Verification items for this drawing (mm, ordinates from the low corner). Round coordinates to 2 decimals unless told otherwise and drop trailing zeros. Order: outer loops, then holes, each group sorted by start corner. A loop starts at its lowest first (then second) coordinate and runs counter-clockwise, first axis right, second up. Notation, with made-up numbers: (-31, 11) - (-7, 11) arc R18 ccw to (-7, 26) - close; hole circle Ø8 at (59, 48). An arc over 180 degrees is marked (long way). Answer as CSV lines item,"result". Start each with the question number.
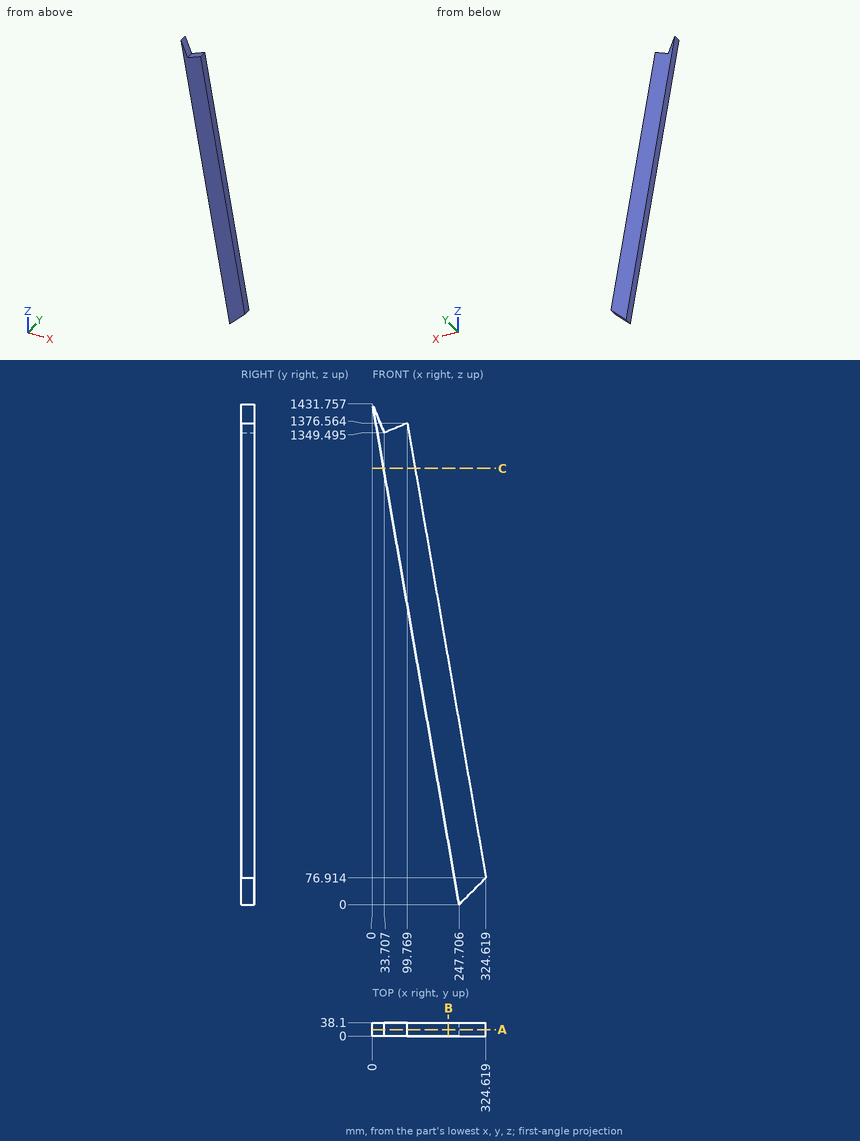
1. Section check A-A on y = 18. Record the boundary of the cut face in (x, z) (1 decimal).
2. Section check B-B on x = 217.5. Record the boundary of the cut face in (y, z).
3. Go/stop test with flat-tipped pins: pin 1 Ø10 at (y, z) = (13, 1215) entering from -X (1 decimal); pin 2 Ø6 at (x, y) = (271.5, 7.5) entering from -Z (1 decimal); pin 3 Ø10 at (y, z) = (21, 1080.5) entering from +X; pin 4 Ø1.5 at (x, z) = (242.5, 446) entering from -Y. Record where each tip stops, or that it passes through.
4. Thickness scan on probe 1 along X at (y, z) = (24.5, 1000); probe 2 along X at (y, z) = (32, 757.5). Record the ranges inside material, lowest first.
5. Section check C-C on z = 1248. Record the boundary of the cut face in (x, y), plus the area to 3 significant figures.
Numbers:
1,outline,"(0, 1431.8) - (247.7, 0) - (324.6, 76.9) - (99.8, 1376.6) - (33.7, 1349.5) - close"
2,outline,"(0, 174.59) - (38.1, 174.59) - (38.1, 696.07) - (0, 696.07) - close"
3,pin 1,"stops at x = 36.6"
3,pin 2,"stops at z = 20.8"
3,pin 3,"stops at x = 151.86"
3,pin 4,"stops at y = 0"
4,probe 1,"x = 74.7 to 164.92"
4,probe 2,"x = 116.65 to 206.87"
5,outline,"(31.79, 0) - (122.01, 0) - (122.01, 38.1) - (31.79, 38.1) - close"
5,area,"3,440 mm2"
